from build123d import *

# Parameters (mm, degrees)
BOSS_EXTRUDE1_DEPTH = 2
SKETCH2_R           = 10
BOSS_EXTRUDE2_DEPTH = 10
SKETCH3_R           = 9
CUT_EXTRUDE1_DEPTH  = 8


with BuildPart() as part:
    # Sketch1 → Boss-Extrude1 (new body)
    with BuildSketch(Plane(origin=(0, 0, 0), x_dir=(1, 0, 0), z_dir=(0, 1, 0))):
        with BuildLine():
            Line((-30, -10), (70, -10))
            ThreePointArc((70, -10), (80, 0), (70, 10))
            Line((70, 10), (-30, 10))
            ThreePointArc((-30, 10), (-40, 0), (-30, -10))
        make_face()
    extrude(amount=BOSS_EXTRUDE1_DEPTH)

    # Sketch2 → Boss-Extrude2 (add)
    with BuildSketch(Plane(origin=(0, 2, 0), x_dir=(1, 0, 0), z_dir=(0, 1, 0))):
        with Locations(Location((-25, 0, 0), (0, 0, 270))):
            Circle(SKETCH2_R)
    extrude(amount=BOSS_EXTRUDE2_DEPTH)

    # Sketch3 → Cut-Extrude1 (cut)
    with BuildSketch(Plane(origin=(0, 12, 0), x_dir=(1, 0, 0), z_dir=(0, 1, 0))):
        with Locations(Location((-25, 0, 0), (0, 0, 270))):
            Circle(SKETCH3_R)
    extrude(amount=-CUT_EXTRUDE1_DEPTH, mode=Mode.SUBTRACT)


solid = part.part
Can you work these out from the model? Positions are in its coordinate system, mm. A direction names the side the tool comes from. Round coordinates to 2 decimals unless told otherwise and drop trailing zeros. Write each loop counter-clockwise with the first axis right and the second up, starting at its lowest first coordinate (ties: lowest second). Pieces come first, ordered by that corner, then holes. Notation, with made-up numbers: M 12,22.25 L 34,22.25 A22 ccw 34,31.25 Z; hole C 13.25,7 d9. An arc over 180 degrees is marked long. Use a Markdown table: item, result.
Item 1: I want a section at C-C (z = -6). List the corners of the cut face in (x, y) for me.
Found:
| item | result |
|---|---|
| outline | M -38,0 L 78,0 L 78,2 L -17,2 L -17,12 L -18.29,12 L -18.29,4 L -31.71,4 L -31.71,12 L -33,12 L -33,2 L -38,2 Z |
Item 2: I want a section at B-B (x = 62.5). List the corners of the cut face in (y, z) for me, and give its area (3 significant figures).
Found:
| item | result |
|---|---|
| outline | M 0,-10 L 2,-10 L 2,10 L 0,10 Z |
| area | 40.0 mm2 |
Item 3: For pin 1 Ø5.5 at (x, z) = (-28.5, -4) entering from +Y; pin 2 Ø5 at (y, z) = (10, 1) entering from -X; pin 3 Ø6 at (x, z) = (48, 2) entering from +Y, each with a flat end and sliding along its axis, tell me the tip position at first contact or that it passes through.
Found:
| item | result |
|---|---|
| pin 1 | stops at y = 4 |
| pin 2 | stops at x = -35 |
| pin 3 | stops at y = 2 |
Item 4: If I drill on line 1 along X through (y, z) = (9.5, 0); line 2 along Y through (x, z) = (-26, -1.75); line 3 along Y through (x, z) = (6.5, 9.25), over which ranges is the centre line in solid material (lowest first)? Write a range as [from, to].
Found:
| item | result |
|---|---|
| line 1 | x = [-35, -34], [-16, -15] |
| line 2 | y = [0, 4] |
| line 3 | y = [0, 2] |
Item 5: We'd pull the mould along Z, two halves only. Please class faces 3 (the face through (-25, 4, 0)), 4 (the face through (-35.3, 2, 0.7)), 5 (the face through (-15.085, 6.93, -1.302)): released by +Z, released by -Z, zero draft, split by the parting line, or undercut.
Found:
| item | result |
|---|---|
| face 3 | undercut |
| face 4 | zero draft |
| face 5 | split by the parting line |
Item 6: Which directions (+Z, -Z, +X, -X, +Y, -Y) give clear straight access to the entire face, cutting with the end or side of a thin tool? Please do faces 1 (the face through (-16.077, 8.056, -1.172)), 2 (the face through (19, 0, 0)).
Found:
| item | result |
|---|---|
| face 1 | +Y |
| face 2 | +Z, -Z, +X, -X, -Y |
Item 7: I want a section at A-A (z = 0). List the corners of the cut face in (x, y) for me.
Found:
| item | result |
|---|---|
| outline | M -40,0 L 80,0 L 80,2 L -15,2 L -15,12 L -16,12 L -16,4 L -34,4 L -34,12 L -35,12 L -35,2 L -40,2 Z |
